Read the model definition and answer for the solid it produces. Units are mm, in the model's axes. Face numbers are marked on the shaded views. Coordinates: 2 decimals unless noted, no trailing zeros. Write each loop counter-clockwise with the first axis right and the second up, starting at its lowest first coordinate (ties: lowest second). Pieces come first, ordered by that corner, then holes. Notation, with made-up numbers: (75.25, 78) - (79.25, 78) arc R27 ccw to (79.25, 106) - close; hole circle Ø11 at (33.5, 32). An arc over 180 degrees is marked (long way). Use a Markdown table: item, result.
from build123d import *


with BuildPart() as part:
    # Sketch2 → Revolve1 (revolve)
    with BuildSketch(Plane.XY, mode=Mode.PRIVATE) as revolve1_sk:
        with BuildLine():
            Line((-6, 6), (-6, 81))
            Line((-6, 81), (-6, 82))
            Line((-6, 82), (-9, 82))
            Line((-9, 82), (-9, 81))
            Line((-9, 81), (-8, 81))
            Line((-8, 81), (-8, 6))
            ThreePointArc((-8, 6), (-5.656854249, 0.343145751), (0, -2))
            Line((0, -2), (0, 0))
            ThreePointArc((0, 0), (-4.242640687, 1.757359313), (-6, 6))
        make_face()
    revolve(revolve1_sk.sketch.rotate(Axis((0, 0, 0), (0, 1, 0)), 270), axis=Axis((0, 0, 0), (0, 1, 0)))


solid = part.part
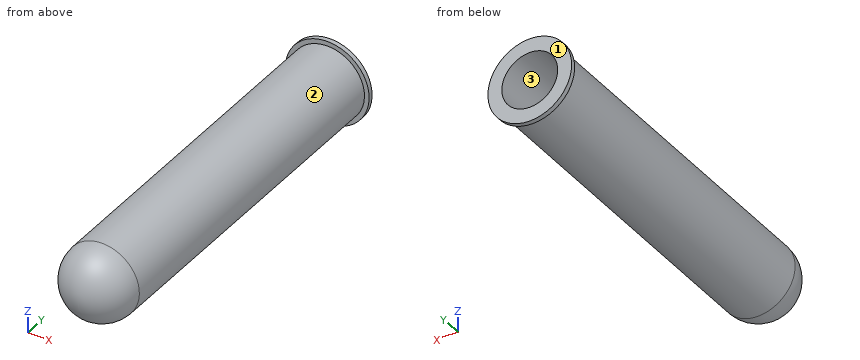
(1) A cutting plane is placed at B-B, the plane z = 0. Write down the section's boundary in (x, y), and give its area (3 significant figures).
Report:
| item | result |
|---|---|
| outline | (-9, 81) - (-8, 81) - (-8, 6) arc R8 ccw to (8, 6) - (8, 81) - (9, 81) - (9, 82) - (6, 82) - (6, 6) arc R6 cw to (-6, 6) - (-6, 82) - (-9, 82) - close |
| area | 350 mm² |
(2) Each of these flat-tipped pins is pushed along its axis until it touches: P1, Ø5, axis at x = 4, z = -3.5, coming from the -Y side; P2, Ø2, axis at x = -0.5, y = 36.5, coming from the -Z side; P3, Ø4, axis at y = 52, z = 0.5, coming from the -X side. Where does it stop, or does it pass through?
Report:
| item | result |
|---|---|
| P1 | stops at y = -1.49 |
| P2 | stops at z = -8 |
| P3 | stops at x = -8 |
(3) A cutting plane is placed at A-A, the plane x = 0. Write down the section's boundary in (y, z), and give its area (3 significant figures).
Report:
| item | result |
|---|---|
| outline | (6, -8) - (81, -8) - (81, -9) - (82, -9) - (82, -6) - (6, -6) arc R6 cw to (6, 6) - (82, 6) - (82, 9) - (81, 9) - (81, 8) - (6, 8) arc R8 ccw to start |
| area | 350 mm² |
(4) Straight lines are drawn through the part: L1, parallel to X at y = 45, z = 0; L2, parallel to Z at x = 0.25, y = 29; L3, parallel to X at y = 41, z = 1. For each, find the intervals that lie inside material, in ascending order.
Report:
| item | result |
|---|---|
| L1 | x = -8 to -6, 6 to 8 |
| L2 | z = -8 to -5.99, 5.99 to 8 |
| L3 | x = -7.94 to -5.92, 5.92 to 7.94 |
(5) The mould has two halves that part along Z. Classify the marked faces 1, 2 and 3: pulls with the +Z half, pulls with the -Z half, needs draft (parallel to the pull), parting line crosses it, or undercut.
Report:
| item | result |
|---|---|
| face 1 | needs draft |
| face 2 | parting line crosses it |
| face 3 | undercut |
(6) A cutting plane is placed at C-C, the plane y = 67.5. Write down the section's boundary in (x, z), and give its area (3 significant figures).
Report:
| item | result |
|---|---|
| outline | circle Ø16 at (0, 0); hole circle Ø12 at (0, 0) |
| area | 88.0 mm² |
